Verification items for the finished model (mm, model axes). A direction names the side the tool comes from. Coordinates: 2 decimals unless noted, no trailing zeros. Loops run counter-clockwise (first coordinate to the right, second up) from the corner with the lowest first, then second, coordinate; pieces in that order, holes last. Notation, with made-up numbers: (49, 86.25) -> (108, 86.25) arc R22 cw to (108, 118.25) -> close; hole circle Ø10 at (1.25, -25). An arc over 180 degrees is marked (long way). Write item = value, one per line.
```python
from build123d import *

# Parameters (mm, degrees)
SKETCH002_W      = 150
SKETCH002_H      = 70
PAD002_DEPTH     = 3
PAD003_DEPTH     = 3
HOLE_D           = 3
HOLE_DEPTH       = 25
HOLE_CSINK_D     = 6.1
HOLE_CSINK_ANGLE = 90
FILLET001_R      = 5
SKETCH009_R      = 6
SKETCH009_R_2    = 3.15
SKETCH009_R_3    = 2
POCKET003_DEPTH  = 5


with BuildPart() as part:
    # Sketch002 → Pad002 (new body)
    with BuildSketch(Plane.XY.offset(41)):
        Rectangle(SKETCH002_W, SKETCH002_H)
    extrude(amount=PAD002_DEPTH)

    # Sketch003 (on Face5 of Pad002) → Pad003 (join)
    with BuildSketch(Plane(origin=(0, 0, 41), x_dir=(1, 0, 0), z_dir=(0, 0, -1))):
        with BuildLine():
            Line((-66.205267, 31.8), (66.205267, 31.8))
            ThreePointArc((66.205267, 31.8), (66.043926, 28.589511), (68.2, 26.205267))
            Line((68.2, -26.205267), (68.2, 26.205267))
            ThreePointArc((68.2, -26.205267), (66.043926, -28.589511), (66.205267, -31.8))
            Line((-66.205267, -31.8), (66.205267, -31.8))
            ThreePointArc((-66.205267, -31.8), (-67.030152, -27.030152), (-71.8, -26.205267))
            Line((-71.8, 26.205267), (-71.8, -26.205267))
            ThreePointArc((-71.8, 26.205267), (-67.030152, 27.030152), (-66.205267, 31.8))
        make_face()
        with BuildLine():
            Line((-62.900704, 28.8), (62.900704, 28.8))
            ThreePointArc((62.900704, 28.8), (63.696162, 26.521261), (65.2, 24.633437))
            Line((65.2, 24.633437), (65.2, -24.633437))
            ThreePointArc((65.2, -24.633437), (63.696162, -26.521261), (62.900704, -28.8))
            Line((62.900704, -28.8), (-62.900704, -28.8))
            ThreePointArc((-62.900704, -28.8), (-64.908831, -24.908831), (-68.8, -22.900704))
            Line((-68.8, -22.900704), (-68.8, 22.900704))
            ThreePointArc((-68.8, 22.900704), (-64.908831, 24.908831), (-62.900704, 28.8))
        make_face(mode=Mode.SUBTRACT)
    extrude(amount=PAD003_DEPTH)

    # Hole
    with Locations(Plane.XY.offset(44)):
        with Locations((-70, 30), (70, 30), (70, -30), (-70, -30)):
            CounterSinkHole(HOLE_D / 2, HOLE_CSINK_D / 2, depth=HOLE_DEPTH, counter_sink_angle=HOLE_CSINK_ANGLE)

    # Fillet001
    fillet001_edges = [part.edges().sort_by_distance(p)[0] for p in [
        (-75, -35, 42.5),
        (75, -35, 42.5),
        (-75, 35, 42.5),
        (75, 35, 42.5),
    ]]
    fillet(fillet001_edges, radius=FILLET001_R)

    # Sketch009 (on Face5 of Fillet001) → Pocket003 (cut)
    with BuildSketch(Plane.XY.offset(44)):
        with Locations((40, -15)):
            Circle(SKETCH009_R)
        with Locations((-40, -15)):
            Circle(SKETCH009_R)
        with Locations((0, -9)):
            Circle(SKETCH009_R_2)
        with Locations((0, -21)):
            Circle(SKETCH009_R_2)
        with Locations((53, 22.5)):
            Circle(SKETCH009_R_3)
    extrude(amount=-POCKET003_DEPTH, mode=Mode.SUBTRACT)


solid = part.part
```
1) Sectioned sample at C-C, the plane z = 39.4. Record the cut outline in (x, y).
Ans:
outline = (-71.8, -26.21) arc R4.2 cw to (-66.21, -31.8) -> (66.21, -31.8) arc R4.2 cw to (68.2, -26.21) -> (68.2, 26.21) arc R4.2 cw to (66.21, 31.8) -> (-66.21, 31.8) arc R4.2 cw to (-71.8, 26.21) -> close; hole (-68.8, -22.9) arc R7.2 cw to (-62.9, -28.8) -> (62.9, -28.8) arc R7.2 cw to (65.2, -24.63) -> (65.2, 24.63) arc R7.2 cw to (62.9, 28.8) -> (-62.9, 28.8) arc R7.2 cw to (-68.8, 22.9) -> close
2) Depth check by flat-ended pin: pin 1 Ø8 at (x, y) = (9.5, -14) entering from -Z; pin 2 Ø2.5 at (x, z) = (-0.5, 39) entering from -Y; pin 3 Ø0.9 at (x, z) = (-10.5, 39.5) entering from +Y. Enter the tip coordinate at first touch or a pass-through.
Ans:
pin_1 = 41
pin_2 = -31.8
pin_3 = 31.8
3) Release check for a two-part mould opening along X. For faces 1 (the face through (-1, -35, 42)), 2 (the face through (-74, -33, 43)), 3 (the face through (63.68, -26.55, 39.52)) record: pulls with the +X half, pulls with the -X half, needs draft (parallel to the pull), parting line crosses it, or undercut.
Ans:
face_1 = needs draft
face_2 = pulls with the -X half
face_3 = undercut
4) Material ranges on line 1 (Y direction, x = 70, z = 41.9); line 2 (Y direction, x = 53, z = 41.9); line 3 (Y direction, x = -37, z = 39.05), recorded low to high.
Ans:
line_1 = -35 to -31.5, -28.5 to 28.5, 31.5 to 35
line_2 = -35 to 20.5, 24.5 to 35
line_3 = -31.8 to -28.8, 28.8 to 31.8
5) Sectioned sample at A-A, the plane x = 0. Record the cut outline in (y, z).
Ans:
outline = (-35, 41) -> (-31.8, 41) -> (-31.8, 38) -> (-28.8, 38) -> (-28.8, 41) -> (-24.15, 41) -> (-24.15, 44) -> (-35, 44) -> close; (-17.85, 41) -> (-12.15, 41) -> (-12.15, 44) -> (-17.85, 44) -> close; (-5.85, 41) -> (28.8, 41) -> (28.8, 38) -> (31.8, 38) -> (31.8, 41) -> (35, 41) -> (35, 44) -> (-5.85, 44) -> close
6) Sectioned sample at D-D, the plane x = 40. Record the cut outline in (y, z).
Ans:
outline = (-35, 41) -> (-31.8, 41) -> (-31.8, 38) -> (-28.8, 38) -> (-28.8, 41) -> (-21, 41) -> (-21, 44) -> (-35, 44) -> close; (-9, 41) -> (28.8, 41) -> (28.8, 38) -> (31.8, 38) -> (31.8, 41) -> (35, 41) -> (35, 44) -> (-9, 44) -> close
7) Sectioned sample at B-B, the plane y = -15. Record the cut outline in (x, z), plus the area to 3 significant figures.
Ans:
outline = (-75, 41) -> (-71.8, 41) -> (-71.8, 38) -> (-68.8, 38) -> (-68.8, 41) -> (-46, 41) -> (-46, 44) -> (-75, 44) -> close; (-34, 41) -> (34, 41) -> (34, 44) -> (-34, 44) -> close; (46, 41) -> (65.2, 41) -> (65.2, 38) -> (68.2, 38) -> (68.2, 41) -> (75, 41) -> (75, 44) -> (46, 44) -> close
area = 396 mm2
8) Tool access check on faces 4 (the face through (-64.953, -24.865, 39.521)), 5 (the face through (68.2, 0, 40)), 6 (the face through (66.06, 28.55, 39.52)). Record the directions out of +Z, -Z, +X, -X, +Y, -Y that give a thin tool (end or side, any length) a straight path to the whole face; none if there is none.
Ans:
face_4 = -Z
face_5 = -Z, +X, +Y, -Y
face_6 = -Z, +X
